The listing builds one solid part. Answer for the finished solid, in the listing's coordinates (mm). Face numbers are marked on the shaded views. A direction names the side the tool comes from. Coordinates: 2 decimals unless noted, no trailing zeros. Loops run counter-clockwise (first coordinate to the right, second up) from the corner with the lowest first, then second, coordinate; pieces in that order, holes last. Notation, with made-up numbers: M 63.25,-2.75 L 92.25,-2.75 A30 cw 92.25,19.25 Z; hole C 27.25,-38 d11. An arc over 180 degrees is marked long. Return JSON: item names as keys, results as strings. Group by question number.
1. Section C-C (x = -1) is taken. Write down the section's boundary in (y, z), then the cut area to 3 significant figures.
2. Section B-B (x = 37) is taken. Write down the section's boundary in (y, z).
3. Straight lines are drawn through the part: L1, parallel to Z at x = -3, y = 2.25; L2, parallel to Y at x = 33.5, z = 0.25; L3, parallel to X at y = -4.25, z = -2. For each, find the intervals that lie inside material, in ascending order. Write a range as from..to.
4. Given P1, Ø1.5, axis at y = -1, z = 5, coming from the +X side; P2, Ø3, axis at y = 5.5, z = -3.5, coming from the -X side; P3, Ø2, axis at x = 6.5, z = -4.5, coming from the -Y side; P4, Ø3, axis at x = -4.5, y = 0.5, coming from the -Z side, each flat-ended and moving along its own axis, determine where each tip first touches the part or whether it passes through.
5. Which of the six approach directions +Z, -Z, +X, -X, +Y, -Y give full straight-line access (tool end or side, diameter ignored) to the marked faces 1, 2 and 3?
6. Section A-A (y = 0) is taken. Write down the section's boundary in (x, z).
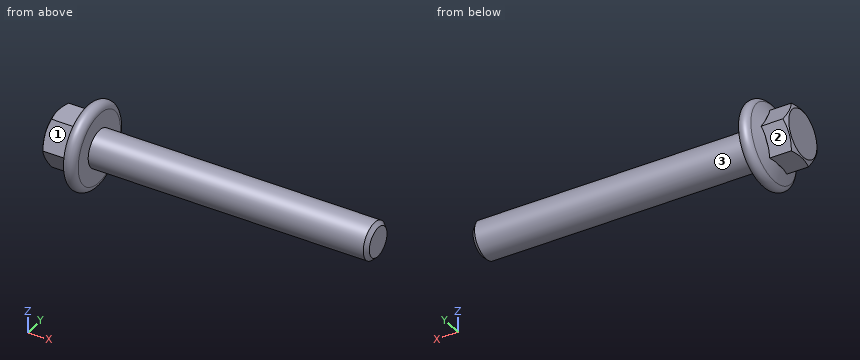
Autodesk Inventor part; units mm, degrees
ref_plane "Work Plane1" through (10.95, 0, 0) normal (0, 0, -1) x (1, 0, 0)
ref_plane "YZ Plane" through (0, 0, 0) normal (1, 0, 0) x (0, 1, 0)
ref_plane "XZ Plane" through (0, 0, 0) normal (0, 1, 0) x (-1, 0, 0)
sketch "Schizzo1" plane through (0, 0, 0) normal (0, 0, 1) x (1, 0, 0)
  line L0 (-3.06, 0) -> (-3.06, 4.0996)
  line L1 (0, 5.7) -> (0, 3)
  line L2 (27, 3) -> (45, 3)
  line L3 (45, 3) -> (45, 0)
  line L4 (45, 0) -> (-3.06, 0)
  arc A0 (0, 5.7) -> (-2.0969, 6.1649) centre (-1.1, 5.7) ccw
  line L5 (0, -1.4013) -> (0, 8.4076)
  line L6 (-12.672, 0) -> (54.612, 0)
  line L7 (0, 3) -> (0.0001, 3)
  line L8 (0.0001, 3) -> (0.0001, 3)
  line L9 (0.0001, 3) -> (26.3865, 3)
  line L10 (26.3865, 3) -> (27, 3)
  line L11 (-3.06, 4.0996) -> (-2.0969, 6.1649)
  line L12 (0.0001, 3) -> (27, 3) construction
  line L13 (27, 3) -> (27, 0) construction
  dimension "d0" = 1.1
  dimension "d1" = 45
  dimension "d2" = 18
  dimension "d3" = 13.6
  dimension "d4" = 6
  dimension "d5" = 3.06
  dimension "d15" = 6
  dimension "d16" = 6
  dimension "d17" = 0.0001
  dimension "d18" = 0.6135
  dimension "d19" = 25
revolve "Corpo" add sketch "Schizzo1" angle 360 about axis through (45, 0, 0) along (-1, 0, 0)
sketch "Schizzo2" plane through (0, 0, 0) normal (1, 0, 0) x (0, 0, -1)
  line L0 (4, 2.3094) -> (4, -2.3094)
  line L1 (4, -2.3094) -> (0, -4.6188)
  line L2 (0, -4.6188) -> (-4, -2.3094)
  line L3 (-4, -2.3094) -> (-4, 2.3094)
  line L4 (-4, 2.3094) -> (0, 4.6188)
  line L5 (0, 4.6188) -> (4, 2.3094)
  point P0 (0, 0)
  point P1 (0, 0)
  dimension "d23" = 8
extrude "Testa" add sketch "Schizzo2" against normal blind 6.8
sketch "Schizzo3" plane through (0, 0, 0) normal (0, 0, 1) x (1, 0, 0)
  line L0 (-6.8, 3.8) -> (-6.8, 4.6188)
  line L1 (-6.8, 4.6188) -> (-6.3273, 4.6188)
  line L2 (-6.3273, 4.6188) -> (-6.8, 3.8)
  line L3 (-7.5964, 0) -> (-2.0215, 0)
  line L4 (-6.8, 4.6188) -> (-6.8, 2.3094)
  line L5 (-2.8179, 4.6188) -> (-6.8, 4.6188)
  point P0 (-6.8, 2.3094)
  dimension "d8" = 30
  dimension "d22" = 7.6
revolve "Smusso1" cut sketch "Schizzo3" angle 360 about axis through (-10, 0, 0) along (1, 0, 0)
thread "Filettatura"
chamfer "Smusso2" distance 0.6135 distance2 0.6135 1 edges at (45, -3, 0) measured on face at (45, 0.3546, -0.711)
ref_plane "Work Plane1" through (10.95, 0, 0) normal (0, 0, -1) x (1, 0, 0)
equation "\"d0\" = PHH"
equation "\"d1\" = NLG"
equation "\"d2\" = GEL"
equation "\"d3\" = LADI"
equation "\"d4\" = GD"
equation "\"d5\" = 0.45 * KOH"
equation "\"d15\" = SD2"
equation "\"d16\" = BDM"
equation "\"d18\" = GAL"
equation "\"d19\" = KEWI"
equation "\"d23\" = SW"
equation "\"d6\" = KOH"
equation "\"d8\" = ANG1"
equation "\"d22\" = SW0"
equation "\"d10\" = GEL"
equation "\"d13\" = -0.5 * SPD + 0.5 * GD"
equation "\"d14\" = GUL"
equation "\"NLG\" = 45"
equation "\"GD\" = NND"
equation "\"BDM\" = NND"
equation "\"KOH\" = 6.8"
equation "\"GEL\" = 18"
equation "\"LADI\" = 13.6"
equation "\"SW\" = 8"
equation "\"PHH\" = RR"
equation "\"SW0\" = 7.6"
equation "\"SPD\" = NND - 1.2269 * PTC"
equation "\"SD2\" = NND"
equation "\"SD\" = 0"
equation "\"ANG1\" = 30deg"
equation "\"KEWI\" = 25deg"
equation "\"GAL\" = 0.61345 * PTC"
equation "\"GUL\" = 0.61345 * PTC"
equation "\"PTC\" = 1"
equation "\"THREADDIA\" = 6"
equation "\"E0\" = 1.155 * SW"
equation "\"TOA\" = 30deg"
equation "\"NND\" = 6"
equation "\"GD1\" = THREADDIA - 1.2269 * PTC"
equation "\"SDH\" = SW"
equation "\"KOH1\" = 2.9"
equation "\"RR\" = 1.1"
properties part number "ISO 4162 - M6 x 45" material "Acciaio inossidabile"
Worked out:
{
 "1": {"outline": "C 0,0 d13.59", "area": "145 mm^2"},
 "2": {"outline": "C 0,0 d6"},
 "3": {"L1": "-4..4", "L2": "-2.99..2.99", "L3": "-2.78..0"},
 "4": {"P1": "x = 0", "P2": "x = -2.63", "P3": "through", "P4": "z = -4.2"},
 "5": {"face 1": "+Z, -X, -Y", "face 2": "-Z, -X, +Y", "face 3": "+X"},
 "6": {"outline": "M -6.8,-3.8 L -6.68,-4 L -3.06,-4 L -3.06,-4.1 L -2.1,-6.16 A1.1 ccw 0,-5.7 L 0,-3 L 44.39,-3 L 45,-2.39 L 45,2.39 L 44.39,3 L 0,3 L 0,5.7 A1.1 ccw -2.1,6.16 L -3.06,4.1 L -3.06,4 L -6.68,4 L -6.8,3.8 Z"}
}
